from build123d import *

# Parameters (mm, degrees)
SKETCH_1_R      = 0.9
EXTRUDE_1_DEPTH = 6
EXTRUDE_2_DEPTH = 3
FILLET_2_R      = 4
FILLET_3_R      = 1
SKETCH_3_R      = 2.5
EXTRUDE_3_DEPTH = 2
FILLET_4_R      = 5
CHAMFER_1_SIZE  = 0.5


with BuildPart() as part:
    # 草图1 → 凸台-拉伸1 (new body)
    with BuildSketch(Plane(origin=(0, 0, 0), x_dir=(1, 0, 0), z_dir=(0, 1, 0))):
        Polygon((0, 12.5), (0, -12.5), (15, -12.5), (15, -8), (12, -5), (12, 5), (15, 8), (15, 12.5), align=None)
        with Locations(Location((5, 3, 0), (0, 0, 270))):
            Circle(SKETCH_1_R, mode=Mode.SUBTRACT)
        with Locations(Location((5, -3, 0), (0, 0, 270))):
            Circle(SKETCH_1_R, mode=Mode.SUBTRACT)
    extrude(amount=EXTRUDE_1_DEPTH)

    # 草图2 → 凸台-拉伸2 (add)
    with BuildSketch(Plane(origin=(0, 6, 0), x_dir=(1, 0, 0), z_dir=(0, 1, 0))):
        with BuildLine():
            Line((13.292893219, 11.792893219), (8, 6.5))
            Line((8, 6.5), (8, -6.5))
            Line((8, -6.5), (13.292893219, -11.792893219))
            ThreePointArc((13.292893219, -11.792893219), (14.382683432, -12.00966597), (15, -11.085786438))
            Line((15, -11.085786438), (15, -8))
            Line((15, -8), (12, -5))
            Line((12, -5), (12, 5))
            Line((12, 5), (15, 8))
            Line((15, 8), (15, 11.085786438))
            ThreePointArc((15, 11.085786438), (14.382683432, 12.00966597), (13.292893219, 11.792893219))
        make_face()
    extrude(amount=EXTRUDE_2_DEPTH)

    # 圆角2
    fillet_2_edges = [part.edges().sort_by_distance(p)[0] for p in [
        (0, 3, 12.5),
        (0, 3, -12.5),
        (8, 7.5, -6.5),
        (8, 7.5, 6.5),
    ]]
    fillet(fillet_2_edges, radius=FILLET_2_R)

    # 圆角3
    fillet_3_edges = [part.edges().sort_by_distance(p)[0] for p in [
        (15, 3, -12.5),
        (15, 3, 12.5),
    ]]
    fillet(fillet_3_edges, radius=FILLET_3_R)

    # 草图3 → 凸台-拉伸3 (add)
    with BuildSketch(Plane(origin=(12, 0, 0), x_dir=(0, 0, -1), z_dir=(1, 0, 0))):
        with Locations(Location((0, 4, 0), (0, 0, 180))):
            Circle(SKETCH_3_R)
    extrude(amount=EXTRUDE_3_DEPTH)

    # 圆角4
    fillet_4_edges = [part.edges().sort_by_distance(p)[0] for p in [
        (15, 4.5, -8),
        (12, 4.5, -5),
        (12, 4.5, 5),
        (15, 4.5, 8),
    ]]
    fillet(fillet_4_edges, radius=FILLET_4_R)

    # 倒角1
    chamfer_1_edges = [part.edges().sort_by_distance(p)[0] for p in [
        (14, 4, -2.5),
    ]]
    chamfer(chamfer_1_edges, length=CHAMFER_1_SIZE)


solid = part.part
For this review, take the finished solid that the model builds, in its own axes (mm). A direction names the side the tool comes from. Round coordinates to 2 decimals unless told otherwise and drop trailing zeros. Order: outer loops, then holes, each group sorted by start corner. A loop starts at its lowest first (then second) coordinate and runs counter-clockwise, first axis right, second up. Notation, with made-up numbers: (10, 85.25) -> (49, 85.25) arc R23 ccw to (49, 120.25) -> close; hole circle Ø4 at (-23, -24). An arc over 180 degrees is marked (long way). Write item = value, one per line. Start each with the question number.
1) Take a section at B-B on y = 0.75. State the section outline as (x, z) points.
2) Tool access review of faces 5 (the face through (8, 7, 0)), 6 (the face through (12.39, 4.56, -4.87)), 7 (the face through (14.367, 7.479, 12.016)): name each direction out of +Z, -Z, +X, -X, +Y, -Y from which nothing blocks a thin tool from reaching the whole face with its end or side.
3) To check wall thickness, follow line 1 (X direction, y = 3.7, z = 3); line 2 (Y direction, x = 3.25, z = 5.25); line 3 (X direction, y = 3.25, z = 1.75). State the ranges of each line that lie inside material, in increasing order. Write a range as from..to.
4) Take a section at D-D on x = 14.25. State the section outline as (y, z) points.
5) Insertion check: pin 1 (1 mm diameter, centred on y = 5.5, z = -1.5, fed in from +X); pin 2 (4 mm diameter, centred on y = 4, z = -5.5, fed in from +X); pin 3 (1.5 mm diameter, centred on y = 1, z = -1, fed in from +X). Each pin has a flat end and moves straight along its axis. Give the tip position at first contact, or say it passes through.
6) The part is to be moulded in two halves that separate along Z. For faces 1 (the face through (7, 0, 0)), 2 (the face through (9, 3, -12.5)), 3 (the face through (12.39, 4.56, 4.87)), 4 (the face through (12, 6.4, 1.3)), say which applies: +Z half, -Z half, draft (parallel to the pull), parting line (faces both ways), or undercut.
7) Take a section at A-A on x = 11.25. State the section outline as (y, z) points.
8) Take a section at C-C on z = 0. State the section outline as (x, y) points.
Verdict:
q1.outline = (0, -8.5) arc R4 ccw to (4, -12.5) -> (14, -12.5) arc R1 ccw to (15, -11.5) -> (15, -10.07) arc R5 ccw to (13.54, -6.54) -> (13.46, -6.46) arc R5 cw to (12, -2.93) -> (12, 2.93) arc R5 cw to (13.46, 6.46) -> (13.54, 6.54) arc R5 ccw to (15, 10.07) -> (15, 11.5) arc R1 ccw to (14, 12.5) -> (4, 12.5) arc R4 ccw to (0, 8.5) -> close; hole circle Ø1.8 at (5, -3); hole circle Ø1.8 at (5, 3)
q2.face_5 = +Z, -Z, -X, +Y
q2.face_6 = +X, +Y, -Y
q2.face_7 = +Z, +Y
q3.line_1 = 0..4.1, 5.9..12
q3.line_2 = 0..6
q3.line_3 = 0..14
q4.outline = (0, -12.47) -> (6, -12.47) -> (6, -12.05) -> (9, -12.05) -> (9, -7.44) -> (0, -7.44) -> close; (0, 7.44) -> (9, 7.44) -> (9, 12.05) -> (6, 12.05) -> (6, 12.47) -> (0, 12.47) -> close
q5.pin_1 = 14
q5.pin_2 = 14.29
q5.pin_3 = 13.59
q6.face_1 = draft
q6.face_2 = -Z half
q6.face_3 = undercut
q6.face_4 = undercut
q7.outline = (0, -12.5) -> (6, -12.5) -> (6, -9.75) -> (9, -9.75) -> (9, 9.75) -> (6, 9.75) -> (6, 12.5) -> (0, 12.5) -> close
q8.outline = (0, 0) -> (12, 0) -> (12, 1.5) -> (13.5, 1.5) -> (14, 2) -> (14, 6) -> (13.5, 6.5) -> (12, 6.5) -> (12, 9) -> (8, 9) -> (8, 6) -> (0, 6) -> close
